Input: part model. Units: mm. Frame: model coordinates. Face numbers are marked on the shaded views. A direction names the side the tool comes from. Round coordinates to 2 decimals unless told otherwise and drop trailing zeros. Write each loop counter-clockwise with the first axis right and the second up, starting at its lowest first coordinate (ties: lowest second). Pieces come first, ordered by that corner, then holes. Notation, with made-up numbers: (-29, 34) -> (25, 34) arc R12 cw to (25, 43) -> close; hole circle Ø2 at (77.25, -27.5). An arc over 180 degrees is marked (long way). Use CSV: the item, a comma, the result in double quotes.
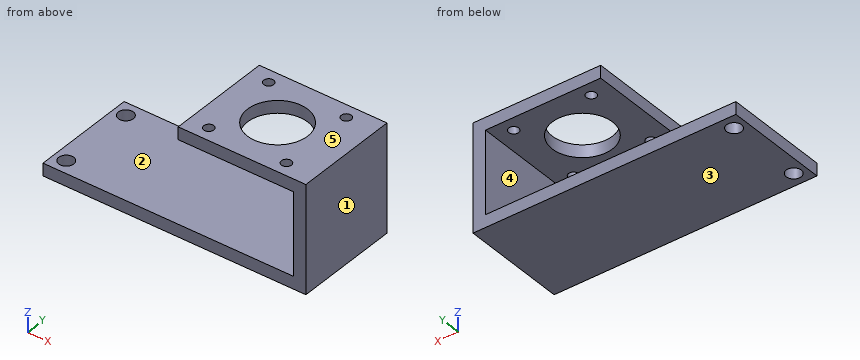
```python
from build123d import *

# Parameters (mm, degrees)
CROQUIS1_W              = 105
CROQUIS1_H              = 42
CROQUIS1_R              = 3
SALIENTE_EXTRUIR1_DEPTH = 5
CROQUIS5_W              = 5
CROQUIS5_H              = 42
SALIENTE_EXTRUIR2_DEPTH = 38
CROQUIS8_W              = 5
CROQUIS8_H              = 42
SALIENTE_EXTRUIR3_DEPTH = 46
CROQUIS10_R             = 2
CROQUIS10_R_2           = 12
CORTAR_EXTRUIR1_DEPTH   = 5


with BuildPart() as part:
    # Croquis1 → Saliente-Extruir1 (new body)
    with BuildSketch(Plane.XY):
        Rectangle(CROQUIS1_W, CROQUIS1_H)
        with Locations((-47.5, 15.44)):
            Circle(CROQUIS1_R, mode=Mode.SUBTRACT)
        with Locations((-47.5, -15.44)):
            Circle(CROQUIS1_R, mode=Mode.SUBTRACT)
    extrude(amount=SALIENTE_EXTRUIR1_DEPTH)

    # Croquis5 → Saliente-Extruir2 (add)
    with BuildSketch(Plane.XY.offset(5)):
        with Locations((50, 0)):
            Rectangle(CROQUIS5_W, CROQUIS5_H)
    extrude(amount=SALIENTE_EXTRUIR2_DEPTH)

    # Croquis8 → Saliente-Extruir3 (add)
    with BuildSketch(Plane.ZY.offset(-47.5)):
        with Locations((40.5, 0)):
            Rectangle(CROQUIS8_W, CROQUIS8_H)
    extrude(amount=SALIENTE_EXTRUIR3_DEPTH)

    # Croquis10 → Cortar-Extruir1 (cut)
    with BuildSketch(Plane.XY.offset(43)):
        with Locations((9.5, 15.5)):
            Circle(CROQUIS10_R)
        with Locations((9.5, -15.5)):
            Circle(CROQUIS10_R)
        with Locations((40.5, -15.5)):
            Circle(CROQUIS10_R)
        with Locations((40.5, 15.5)):
            Circle(CROQUIS10_R)
        with Locations((25, 0)):
            Circle(CROQUIS10_R_2)
    extrude(amount=-CORTAR_EXTRUIR1_DEPTH, mode=Mode.SUBTRACT)


solid = part.part
```
Item 1: Line query: line 1 (Y direction, x = -47.5, z = 3.2); line 2 (Y direction, x = 40.5, z = 41.75); line 3 (Z direction, x = 12, y = 19). Output: solid intervals per line, ascending.
Worked answers:
line 1,"y = -21 to -18.44, -12.44 to 12.44, 18.44 to 21"
line 2,"y = -21 to -17.5, -13.5 to 13.5, 17.5 to 21"
line 3,"z = 0 to 5, 38 to 43"
Item 2: Section query D-D on z = 31.5. Return the cut outline in (x, y).
Worked answers:
outline,"(47.5, -21) -> (52.5, -21) -> (52.5, 21) -> (47.5, 21) -> close"
Item 3: First-contact query: pin 1 Ø4 at (y, z) = (8, 12) entering from -X; pin 2 Ø3.5 at (x, y) = (-47.5, 15.44) entering from -Z; pin 3 Ø5.5 at (y, z) = (0.5, 40) entering from -X. Flat tips, straight axial feed; report the tip coordinate or a pass-through.
Worked answers:
pin 1,"stops at x = 47.5"
pin 2,"passes through"
pin 3,"stops at x = 1.5"
Item 4: Set-up query: the marked faces 4 and 5. Return all of +Z, -Z, +X, -X, +Y, -Y with unobstructed straight access to the full face (end or side cutting, diameter ignored); none if empty.
Worked answers:
face 4,"-X, +Y, -Y"
face 5,"+Z, +X, -X, +Y, -Y"
Item 5: Section query A-A on x = -47.5. Return the cut outline in (y, z), plus the area to 3 significant figures.
Worked answers:
outline,"(-21, 0) -> (-18.44, 0) -> (-18.44, 5) -> (-21, 5) -> close; (-12.44, 0) -> (12.44, 0) -> (12.44, 5) -> (-12.44, 5) -> close; (18.44, 0) -> (21, 0) -> (21, 5) -> (18.44, 5) -> close"
area,"150 mm²"
Item 6: Section query C-C on x = 9.5. Return the cut outline in (y, z).
Worked answers:
outline,"(-21, 0) -> (21, 0) -> (21, 5) -> (-21, 5) -> close; (-21, 38) -> (-17.5, 38) -> (-17.5, 43) -> (-21, 43) -> close; (-13.5, 38) -> (13.5, 38) -> (13.5, 43) -> (-13.5, 43) -> close; (17.5, 38) -> (21, 38) -> (21, 43) -> (17.5, 43) -> close"
Item 7: Pull-direction query (Z, two-part tool) for the marked faces 1, 2 and 3; classes: +Z half, -Z half, draft (parallel to the pull), parting line (faces both ways), or undercut.
Worked answers:
face 1,"draft"
face 2,"undercut"
face 3,"-Z half"
Item 8: Section query B-B on y = 6. Return the cut outline in (x, z), plus the area to 3 significant figures.
Worked answers:
outline,"(-52.5, 0) -> (52.5, 0) -> (52.5, 43) -> (35.39, 43) -> (35.39, 38) -> (47.5, 38) -> (47.5, 5) -> (-52.5, 5) -> close; (1.5, 38) -> (14.61, 38) -> (14.61, 43) -> (1.5, 43) -> close"
area,"841 mm²"
